Model file for the job. Use its own axes, mm. A direction names the side the tool comes from. Coordinates: 2 decimals unless noted, no trailing zeros. Write each loop counter-clockwise with the first axis right and the second up, starting at its lowest first coordinate (ties: lowest second). Pieces come first, ordered by that corner, then holes.
Q1. Band-saw the part on D-D, the plane x = 12.5. Write the cut outline in (y, z).
Q2. Band-saw the part on A-A, the plane x = 0. Write the cut outline in (y, z) (3 decimals), plus the area to 3 significant figures.
Q3. Which spindle directions (+Z, -Z, +X, -X, +Y, -Y) get a long thin tool onto all of the face, cutting with end or side? Do faces 1 (the flat face through (-20, -13, -0.5)), 2 (the flat face through (13.5, -21.3, 0)), 3 (the flat face through (0, 0, 0.5)). Say none if no direction does.
Q4. Pin check, flat tips, straight feed: P1, Ø4.5, axis at x = 20, y = -11, coming from the -Z side; P2, Ø2, axis at x = -19, y = -11, coming from the -Z side; P3, Ø1.5, axis at x = -3.5, z = -1, coming from the -Y side. Stop position of each tip, or through.
Q5. Pull direction Y, two halves, no side cores. Call faces 4 (the cylindrical face through (23.846, 7.509, 0.246)), 5 (the flat face through (20, -13, -0.5)), 6 (the flat face through (0, 21, -0.5)), 7 (the flat face through (0, 0, -2)): released by +Y, released by -Y, zero draft, split by the parting line, or undercut.
Q6. Drill centre lines: probe 1 along X at (y, z) = (-12, -0.7); probe 2 along Y at (x, z) = (-20.5, 0.15); probe 3 along X at (y, z) = (21.5, -1.65). Where is each one in solid material? Low to high.
Q7. Band-saw the part on B-B, the plane z = -1.2. Write the cut outline in (x, y) (3 decimals).
Q8. Band-saw the part on C-C, the plane y = 15. Write the cut outline in (x, z).
from build123d import *
from build123d import SkipClean  # not in build123d's __all__

# Parameters (mm, degrees)
F0_R     = 25
F1_DEPTH = 0.5
F0_R_2   = 26.25
F2_DEPTH = 2
F3_DEPTH = 0.5


with BuildPart() as f1:
    # F0 (on Top) → F1 (new body)
    with BuildSketch(Plane.XY):
        Circle(F0_R)
        with BuildLine():
            ThreePointArc((1.998066932, 22.6620879121), (16.7782377308, 15.3640241684), (22.75, 0))
            ThreePointArc((22.75, 0), (22.2123921898, -4.9165163688), (20.6249773007, -9.6006672345))
            ThreePointArc((20.6249773007, -9.6006672345), (21.4117268371, -10.3371654104), (21.7020779361, -11.375))
            ThreePointArc((21.7020779361, -11.375), (20.6637600211, -13.12861557), (18.6269103687, -13.0614206776))
            ThreePointArc((18.6269103687, -13.0614206776), (0, -22.75), (-18.6269103687, -13.0614206776))
            ThreePointArc((-18.6269103687, -13.0614206776), (-21.4341287437, -12.375), (-20.6249773007, -9.6006672345))
            ThreePointArc((-20.6249773007, -9.6006672345), (-19.7020779361, 11.375), (-1.998066932, 22.6620879121))
            ThreePointArc((-1.998066932, 22.6620879121), (-0.0439666691, 24.7495166746), (2, 22.75))
            ThreePointArc((2, 22.75), (1.9995166746, 22.7060333309), (1.998066932, 22.6620879121))
        make_face(mode=Mode.SUBTRACT)
        with BuildLine():
            ThreePointArc((20.6249773007, -9.6006672345), (22.2123921898, -4.9165163688), (22.75, 0))
            ThreePointArc((22.75, 0), (16.7782377308, 15.3640241684), (1.998066932, 22.6620879121))
            ThreePointArc((1.998066932, 22.6620879121), (0, 20.75), (-1.998066932, 22.6620879121))
            ThreePointArc((-1.998066932, 22.6620879121), (-19.7020779361, 11.375), (-20.6249773007, -9.6006672345))
            ThreePointArc((-20.6249773007, -9.6006672345), (-18.6642433465, -9.665351099), (-17.7020779361, -11.375))
            ThreePointArc((-17.7020779361, -11.375), (-17.9484623661, -12.336682085), (-18.6269103687, -13.0614206776))
            ThreePointArc((-18.6269103687, -13.0614206776), (0, -22.75), (18.6269103687, -13.0614206776))
            ThreePointArc((18.6269103687, -13.0614206776), (17.9700271285, -10.375), (20.6249773007, -9.6006672345))
        make_face()
        with BuildLine():
            ThreePointArc((-20.3083862198, -10.2533872036), (-20.4692836493, -9.9282892225), (-20.6249773007, -9.6006672345))
            ThreePointArc((-20.6249773007, -9.6006672345), (-21.4341287437, -12.375), (-18.6269103687, -13.0614206776))
            ThreePointArc((-18.6269103687, -13.0614206776), (-18.8327925074, -12.7627750263), (-19.0338869031, -12.4608847744))
            ThreePointArc((-19.0338869031, -12.4608847744), (-20.8062603259, -12.0125), (-20.3083862198, -10.2533872036))
        make_face()
        with BuildLine():
            ThreePointArc((21.7020779361, -11.375), (21.4117268371, -10.3371654104), (20.6249773007, -9.6006672345))
            ThreePointArc((20.6249773007, -9.6006672345), (20.4692836493, -9.9282892225), (20.3083862198, -10.2533872036))
            ThreePointArc((20.3083862198, -10.2533872036), (20.797219037, -10.7220903821), (20.9770779361, -11.375))
            ThreePointArc((20.9770779361, -11.375), (20.3240431413, -12.4880068659), (19.0338869031, -12.4608847744))
            ThreePointArc((19.0338869031, -12.4608847744), (18.8327925074, -12.7627750263), (18.6269103687, -13.0614206776))
            ThreePointArc((18.6269103687, -13.0614206776), (20.6637600211, -13.12861557), (21.7020779361, -11.375))
        make_face()
        with BuildLine():
            ThreePointArc((1.2744993168, 22.714271978), (1.6364911418, 22.6910642488), (1.998066932, 22.6620879121))
            ThreePointArc((1.998066932, 22.6620879121), (1.9995166746, 22.7060333309), (2, 22.75))
            ThreePointArc((2, 22.75), (-0.0439666691, 24.7495166746), (-1.998066932, 22.6620879121))
            ThreePointArc((-1.998066932, 22.6620879121), (-1.6364911418, 22.6910642488), (-1.2744993168, 22.714271978))
            ThreePointArc((-1.2744993168, 22.714271978), (-0.017865765, 24.024874823), (1.275, 22.75))
            ThreePointArc((1.275, 22.75), (1.274874823, 22.732134235), (1.2744993168, 22.714271978))
        make_face()
        with BuildLine():
            ThreePointArc((-17.7020779361, -11.375), (-18.6642433465, -9.665351099), (-20.6249773007, -9.6006672345))
            ThreePointArc((-20.6249773007, -9.6006672345), (-20.4692836493, -9.9282892225), (-20.3083862198, -10.2533872036))
            ThreePointArc((-20.3083862198, -10.2533872036), (-19.0491683182, -10.2798588991), (-18.4270779361, -11.375))
            ThreePointArc((-18.4270779361, -11.375), (-18.5890710702, -11.9969652052), (-19.0338869031, -12.4608847744))
            ThreePointArc((-19.0338869031, -12.4608847744), (-18.8327925074, -12.7627750263), (-18.6269103687, -13.0614206776))
            ThreePointArc((-18.6269103687, -13.0614206776), (-17.9484623661, -12.336682085), (-17.7020779361, -11.375))
        make_face()
        with BuildLine():
            ThreePointArc((20.3083862198, -10.2533872036), (20.4692836493, -9.9282892225), (20.6249773007, -9.6006672345))
            ThreePointArc((20.6249773007, -9.6006672345), (17.9700271285, -10.375), (18.6269103687, -13.0614206776))
            ThreePointArc((18.6269103687, -13.0614206776), (18.8327925074, -12.7627750263), (19.0338869031, -12.4608847744))
            ThreePointArc((19.0338869031, -12.4608847744), (18.5978955463, -10.7375), (20.3083862198, -10.2533872036))
        make_face()
        with BuildLine():
            ThreePointArc((-1.998066932, 22.6620879121), (0, 20.75), (1.998066932, 22.6620879121))
            ThreePointArc((1.998066932, 22.6620879121), (1.6364911418, 22.6910642488), (1.2744993168, 22.714271978))
            ThreePointArc((1.2744993168, 22.714271978), (0, 21.475), (-1.2744993168, 22.714271978))
            ThreePointArc((-1.2744993168, 22.714271978), (-1.6364911418, 22.6910642488), (-1.998066932, 22.6620879121))
        make_face()
    extrude(amount=F1_DEPTH)

    # F0 (on Top) → F2 (join)
    with BuildSketch(Plane.XY):
        Circle(F0_R_2)
        Circle(F0_R, mode=Mode.SUBTRACT)
        Circle(F0_R)
        with BuildLine():
            ThreePointArc((1.998066932, 22.6620879121), (16.7782377308, 15.3640241684), (22.75, 0))
            ThreePointArc((22.75, 0), (22.2123921898, -4.9165163688), (20.6249773007, -9.6006672345))
            ThreePointArc((20.6249773007, -9.6006672345), (21.4117268371, -10.3371654104), (21.7020779361, -11.375))
            ThreePointArc((21.7020779361, -11.375), (20.6637600211, -13.12861557), (18.6269103687, -13.0614206776))
            ThreePointArc((18.6269103687, -13.0614206776), (0, -22.75), (-18.6269103687, -13.0614206776))
            ThreePointArc((-18.6269103687, -13.0614206776), (-21.4341287437, -12.375), (-20.6249773007, -9.6006672345))
            ThreePointArc((-20.6249773007, -9.6006672345), (-19.7020779361, 11.375), (-1.998066932, 22.6620879121))
            ThreePointArc((-1.998066932, 22.6620879121), (-0.0439666691, 24.7495166746), (2, 22.75))
            ThreePointArc((2, 22.75), (1.9995166746, 22.7060333309), (1.998066932, 22.6620879121))
        make_face(mode=Mode.SUBTRACT)
        with BuildLine():
            ThreePointArc((20.6249773007, -9.6006672345), (22.2123921898, -4.9165163688), (22.75, 0))
            ThreePointArc((22.75, 0), (16.7782377308, 15.3640241684), (1.998066932, 22.6620879121))
            ThreePointArc((1.998066932, 22.6620879121), (0, 20.75), (-1.998066932, 22.6620879121))
            ThreePointArc((-1.998066932, 22.6620879121), (-19.7020779361, 11.375), (-20.6249773007, -9.6006672345))
            ThreePointArc((-20.6249773007, -9.6006672345), (-18.6642433465, -9.665351099), (-17.7020779361, -11.375))
            ThreePointArc((-17.7020779361, -11.375), (-17.9484623661, -12.336682085), (-18.6269103687, -13.0614206776))
            ThreePointArc((-18.6269103687, -13.0614206776), (0, -22.75), (18.6269103687, -13.0614206776))
            ThreePointArc((18.6269103687, -13.0614206776), (17.9700271285, -10.375), (20.6249773007, -9.6006672345))
        make_face()
    extrude(amount=-F2_DEPTH)

    # F0 (on Top) → F3 (join)
    with BuildSketch(Plane.XY):
        with BuildLine():
            ThreePointArc((1.2744993168, 22.714271978), (1.6364911418, 22.6910642488), (1.998066932, 22.6620879121))
            ThreePointArc((1.998066932, 22.6620879121), (1.9995166746, 22.7060333309), (2, 22.75))
            ThreePointArc((2, 22.75), (-0.0439666691, 24.7495166746), (-1.998066932, 22.6620879121))
            ThreePointArc((-1.998066932, 22.6620879121), (-1.6364911418, 22.6910642488), (-1.2744993168, 22.714271978))
            ThreePointArc((-1.2744993168, 22.714271978), (-0.017865765, 24.024874823), (1.275, 22.75))
            ThreePointArc((1.275, 22.75), (1.274874823, 22.732134235), (1.2744993168, 22.714271978))
        make_face()
        with BuildLine():
            ThreePointArc((-1.998066932, 22.6620879121), (0, 20.75), (1.998066932, 22.6620879121))
            ThreePointArc((1.998066932, 22.6620879121), (1.6364911418, 22.6910642488), (1.2744993168, 22.714271978))
            ThreePointArc((1.2744993168, 22.714271978), (0, 21.475), (-1.2744993168, 22.714271978))
            ThreePointArc((-1.2744993168, 22.714271978), (-1.6364911418, 22.6910642488), (-1.998066932, 22.6620879121))
        make_face()
        with BuildLine():
            ThreePointArc((-20.3083862198, -10.2533872036), (-20.4692836493, -9.9282892225), (-20.6249773007, -9.6006672345))
            ThreePointArc((-20.6249773007, -9.6006672345), (-21.4341287437, -12.375), (-18.6269103687, -13.0614206776))
            ThreePointArc((-18.6269103687, -13.0614206776), (-18.8327925074, -12.7627750263), (-19.0338869031, -12.4608847744))
            ThreePointArc((-19.0338869031, -12.4608847744), (-20.8062603259, -12.0125), (-20.3083862198, -10.2533872036))
        make_face()
        with BuildLine():
            ThreePointArc((-17.7020779361, -11.375), (-18.6642433465, -9.665351099), (-20.6249773007, -9.6006672345))
            ThreePointArc((-20.6249773007, -9.6006672345), (-20.4692836493, -9.9282892225), (-20.3083862198, -10.2533872036))
            ThreePointArc((-20.3083862198, -10.2533872036), (-19.0491683182, -10.2798588991), (-18.4270779361, -11.375))
            ThreePointArc((-18.4270779361, -11.375), (-18.5890710702, -11.9969652052), (-19.0338869031, -12.4608847744))
            ThreePointArc((-19.0338869031, -12.4608847744), (-18.8327925074, -12.7627750263), (-18.6269103687, -13.0614206776))
            ThreePointArc((-18.6269103687, -13.0614206776), (-17.9484623661, -12.336682085), (-17.7020779361, -11.375))
        make_face()
        with BuildLine():
            ThreePointArc((20.3083862198, -10.2533872036), (20.4692836493, -9.9282892225), (20.6249773007, -9.6006672345))
            ThreePointArc((20.6249773007, -9.6006672345), (17.9700271285, -10.375), (18.6269103687, -13.0614206776))
            ThreePointArc((18.6269103687, -13.0614206776), (18.8327925074, -12.7627750263), (19.0338869031, -12.4608847744))
            ThreePointArc((19.0338869031, -12.4608847744), (18.5978955463, -10.7375), (20.3083862198, -10.2533872036))
        make_face()
        with BuildLine():
            ThreePointArc((21.7020779361, -11.375), (21.4117268371, -10.3371654104), (20.6249773007, -9.6006672345))
            ThreePointArc((20.6249773007, -9.6006672345), (20.4692836493, -9.9282892225), (20.3083862198, -10.2533872036))
            ThreePointArc((20.3083862198, -10.2533872036), (20.797219037, -10.7220903821), (20.9770779361, -11.375))
            ThreePointArc((20.9770779361, -11.375), (20.3240431413, -12.4880068659), (19.0338869031, -12.4608847744))
            ThreePointArc((19.0338869031, -12.4608847744), (18.8327925074, -12.7627750263), (18.6269103687, -13.0614206776))
            ThreePointArc((18.6269103687, -13.0614206776), (20.6637600211, -13.12861557), (21.7020779361, -11.375))
        make_face()
    with SkipClean():  # cleaning this boolean's faces spoils the solid; the shape is the same uncleaned
        extrude(amount=-F3_DEPTH)


solid = f1.part
Answer sheet:
1. outline: (-23.08, -2) - (23.08, -2) - (23.08, 0) - (21.65, 0) - (21.65, 0.5) - (-21.65, 0.5) - (-21.65, 0) - (-23.08, 0) - close
2. outline: (-26.25, -2) - (20.75, -2) - (20.75, -0.5) - (21.475, -0.5) - (21.475, 0.5) - (-25, 0.5) - (-25, 0) - (-26.25, 0) - close; (24.025, -0.5) - (24.75, -0.5) - (24.75, -2) - (26.25, -2) - (26.25, 0) - (25, 0) - (25, 0.5) - (24.025, 0.5) - close
2. area: 121 mm2
3. face 1: -Z
3. face 2: +Z
3. face 3: +Z, +X, -X, +Y, -Y
4. P1: stops at z = -2
4. P2: stops at z = -0.5
4. P3: stops at y = -26.11
5. face 4: split by the parting line
5. face 5: undercut
5. face 6: undercut
5. face 7: zero draft
6. probe 1: x = -23.35 to -21.6, -17.8 to 17.8, 21.6 to 23.35
6. probe 2: y = -14.31 to -12.37, -10.38 to 14.31
6. probe 3: x = -15.06 to -1.56, 1.56 to 15.06
7. outline: circle Ø52.5 at (0, 0); hole circle Ø4 at (-19.702, -11.375); hole circle Ø4 at (0, 22.75); hole circle Ø4 at (19.702, -11.375)
8. outline: (-21.54, -2) - (21.54, -2) - (21.54, 0) - (20, 0) - (20, 0.5) - (-20, 0.5) - (-20, 0) - (-21.54, 0) - close
